Study the drawing (mm; zero at the part's minimum x, y, z) and answer. A direction names the side the tool comes from. Round coordinates to 2 decimals unless told otherwise and drop trailing zeros. Write each loop counter-clockwise with the first axis right and the second up, starting at its lowest first coordinate (ties: lowest second). Pieces come first, ordered by that corner, then holes. Notation, with made-up numbers: (-37, 10.25) -> (12, 10.25) arc R21 cw to (12, 31.25) -> close; hole circle Ø1 at (2, 57). An arc over 180 degrees is marked (long way). Return JSON: item names as keys, results as strings.
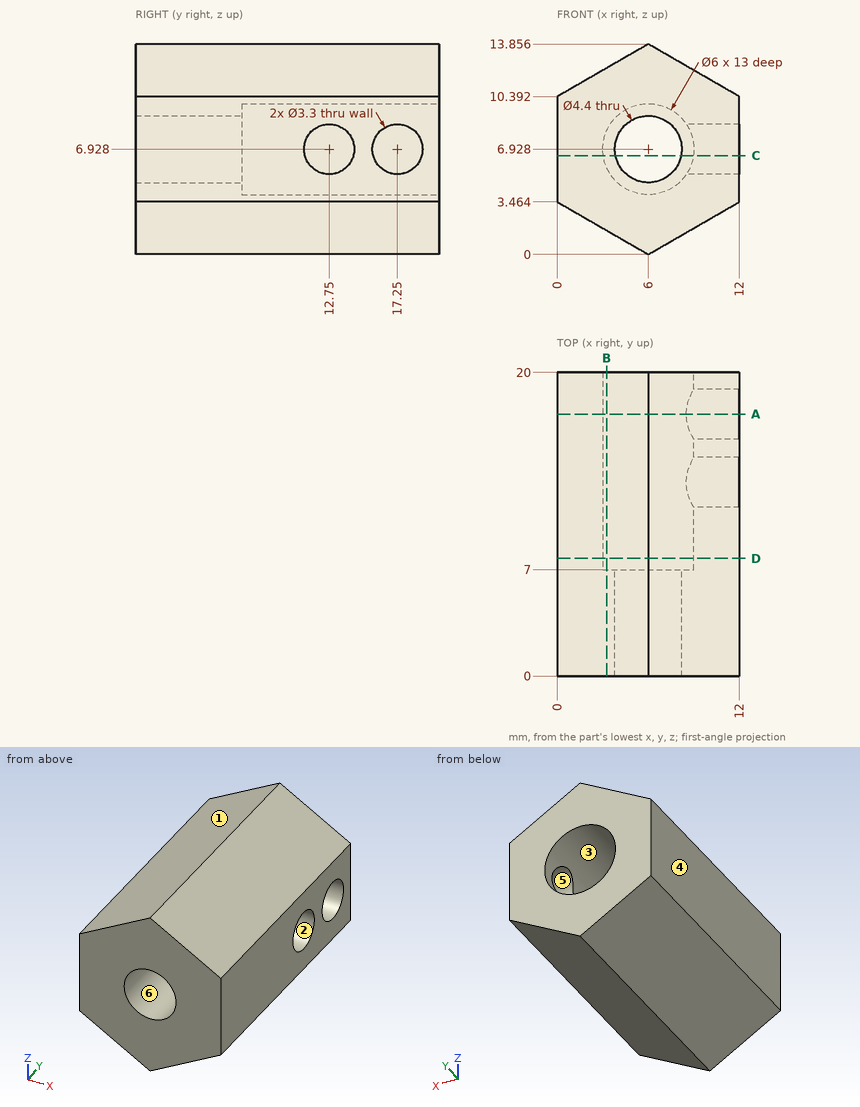
Item 1: Flat-ended cylindrical pins translate along their axes: pin 1 (4 mm diameter, centred on x = 6, y = 7, fed in from +Z); pin 2 (5.5 mm diameter, centred on x = 6, z = 6.93, fed in from +Y); pin 3 (3 mm diameter, centred on y = 12.75, z = 6.93, fed in from +X). Find the tip coordinate at first contact, or state that the pin passes through.
Worked answers:
{"pin 1": "stops at z = 13.86", "pin 2": "stops at y = 7", "pin 3": "stops at x = 3.4"}
Item 2: Section D-D (y = 7.75) is taken. Give the vertices of the cut face in (x, z).
Worked answers:
{"outline": "(0, 3.46) -> (6, 0) -> (12, 3.46) -> (12, 10.39) -> (6, 13.86) -> (0, 10.39) -> close; hole circle Ø6 at (6, 6.93)"}
Item 3: Section B-B (x = 3.25) is taken. Give the vertices of the cut face in (y, z).
Worked answers:
{"outline": "(0, 1.59) -> (20, 1.59) -> (20, 5.73) -> (7, 5.73) -> (7, 8.13) -> (20, 8.13) -> (20, 12.27) -> (0, 12.27) -> close"}
Item 4: Section C-C (z = 6.5) is taken. Give the vertices of the cut face in (x, y).
Worked answers:
{"outline": "(0, 0) -> (3.84, 0) -> (3.84, 7) -> (3.03, 7) -> (3.03, 20) -> (0, 20) -> close; (8.16, 0) -> (12, 0) -> (12, 11.16) -> (8.97, 11.16) -> (8.97, 7) -> (8.16, 7) -> close; (8.97, 14.34) -> (12, 14.34) -> (12, 15.66) -> (8.97, 15.66) -> close; (8.97, 18.84) -> (12, 18.84) -> (12, 20) -> (8.97, 20) -> close"}
Item 5: Straight lines are drawn through the part: L1, parallel to X at y = 10.75, z = 5; L2, parallel to Z at x = 6.75, y = 3.75 (1 decimal); L3, parallel to X at y = 10, z = 6. For each, find the intervals that lie inside material, in ascending order. Write a range as [from, to].
Worked answers:
{"L1": "x = [0, 3.7], [8.3, 12]", "L2": "z = [0.4, 4.9], [9, 13.4]", "L3": "x = [0, 3.15], [8.85, 12]"}
Item 6: A tool of negligible diameter and unlimited length cuts with its end or side. For the marked faces 1, 2 and 3, from which of +Z, -Z, +X, -X, +Y, -Y can it reach the whole face along a straight path? Write none if from no direction.
Worked answers:
{"face 1": "+Z, -X, +Y, -Y", "face 2": "+X", "face 3": "+Y"}
Item 7: For a pull along X with two mould halves and no side action, classify the marked faces 4, 5 and 6 as released by +X, released by -X, zero draft, split by the parting line, or undercut.
Worked answers:
{"face 4": "released by -X", "face 5": "zero draft", "face 6": "undercut"}
Item 8: Section A-A (y = 17.25) is taken. Give the vertices of the cut face in (x, z) (1 decimal).
Worked answers:
{"outline": "(0, 3.5) -> (6, 0) -> (12, 3.5) -> (12, 5.3) -> (8.5, 5.3) arc R3 cw (long way) to (8.5, 8.6) -> (12, 8.6) -> (12, 10.4) -> (6, 13.9) -> (0, 10.4) -> close"}
